Check sheet for the modelled part. Datum: model origin and axes. Units: mm. A direction names the side the tool comes from. Give positions to 0.01 mm unless a question says otherwise; leave off trailing zeros. Order: outer loops, then holes, each group sorted by start corner. A loop starts at its lowest first (then second) coordinate and runs counter-clockwise, first axis right, second up. Notation, with made-up numbers: (75, -1.5) - (97, -1.5) arc R29 ccw to (97, 34.5) - close; hole circle Ø1 at (62, 65.25). An arc over 180 degrees is marked (long way). Answer in a Markdown table with one row per item.
from build123d import *

# Parameters (mm, degrees)
SKETCH1_W                     = 60
SKETCH1_H                     = 60
BOSS_EXTRUDE1_DEPTH           = 10
SKETCH1_3_W                   = 9.5
SKETCH1_3_H                   = 10
BOSS_EXTRUDE2_DEPTH           = 20
BOSS_EXTRUDE3_START           = -10
SKETCH1_4_W                   = 34.6
SKETCH1_4_H                   = 60
BOSS_EXTRUDE3_DEPTH           = 22.5
CBORE_FOR_M3_SHCS1_AT_2_COUNT = 2
CBORE_FOR_M3_SHCS1_AT_2_PITCH = 40
SKETCH6_R                     = 2.25
CUT_EXTRUDE1_DEPTH            = 10
FILLET1_R                     = 1


with BuildPart() as part:
    # Sketch1 → Boss-Extrude1 (new body)
    with BuildSketch(Plane(origin=(0, 0, 0), x_dir=(1, 0, 0), z_dir=(0, 1, 0))):
        Rectangle(SKETCH1_W, SKETCH1_H)
    extrude(amount=-BOSS_EXTRUDE1_DEPTH)

    # Sketch1<3> → Boss-Extrude2 (add)
    with BuildSketch(Plane(origin=(0, 0, 0), x_dir=(1, 0, 0), z_dir=(0, 1, 0))):
        with Locations((-25.25, -15.65)):
            Rectangle(SKETCH1_3_W, SKETCH1_3_H)
        with Locations((25.25, -15.65)):
            Rectangle(SKETCH1_3_W, SKETCH1_3_H)
    extrude(amount=BOSS_EXTRUDE2_DEPTH)

    # Sketch1<4> → Boss-Extrude3 (add)
    with BuildSketch(Plane(origin=(0, 0, 0), x_dir=(1, 0, 0), z_dir=(0, 1, 0)).offset(BOSS_EXTRUDE3_START)):
        with Locations((12.7, 0)):
            Rectangle(SKETCH1_4_W, SKETCH1_4_H)
    extrude(amount=-BOSS_EXTRUDE3_DEPTH)

    # Sketch3 → CBORE for M3 SHCS1 (revolve, cut)
    with BuildSketch(Plane(origin=(30, -23.49, 20), x_dir=(0, 0, -1), z_dir=(0, 1, 0))):
        Polygon((0, 0), (0, 35.681549114), (1.8, 34.6), (1.8, 23), (3.25, 23), (3.25, 0.025), (3.275, 0), align=None)
    cbore_for_m3_shcs1 = revolve(axis=Axis((36.35, -23.49, 20), (-1, 0, 0)), mode=Mode.SUBTRACT)

    # CBORE for M3 SHCS1 at 2: CBORE for M3 SHCS1 ×2
    with Locations(*[(0, 0, -i * CBORE_FOR_M3_SHCS1_AT_2_PITCH) for i in range(1, CBORE_FOR_M3_SHCS1_AT_2_COUNT)]):
        add(cbore_for_m3_shcs1, mode=Mode.SUBTRACT)

    # Sketch5 → CBORE for M3 SHCS2 (revolve, cut)
    with BuildSketch(Plane(origin=(-18.09, 0, -20), x_dir=(0, 0, 1), z_dir=(1, 0, 0))):
        Polygon((0, 0), (0, 11.081549114), (1.8, 10), (1.8, 3), (3.25, 3), (3.25, 0.025), (3.275, 0), align=None)
    revolve(axis=Axis((-18.09, 6.35, -20), (0, -1, 0)), mode=Mode.SUBTRACT)

    # Sketch6 → Cut-Extrude1 (cut)
    with BuildSketch(Plane.XY.offset(20.65)):
        with Locations((-23.725, 15)):
            Circle(SKETCH6_R)
        with Locations((-23.725, 5)):
            Circle(SKETCH6_R)
        with Locations(Location((23.725, 5, 0), (0, 0, 180))):
            Circle(SKETCH6_R)
        with Locations(Location((23.725, 15, 0), (0, 0, 180))):
            Circle(SKETCH6_R)
    extrude(amount=-CUT_EXTRUDE1_DEPTH, mode=Mode.SUBTRACT)

    # Fillet1
    fillet1_edges = [part.edges().sort_by_distance(p)[0] for p in [
        (-17.3, -10, -30),
        (-30, -10, 0),
        (-30, 0, 25.325),
        (-25.25, 20, 20.65),
        (-30, 10, 20.65),
        (-20.5, 20, 15.65),
        (-25.25, 20, 10.65),
        (-30, 10, 10.65),
        (-30, 20, 15.65),
        (-25.25, 0, 20.65),
        (-25.25, 0, 10.65),
        (30, 0, 25.325),
        (30, 20, 15.65),
        (30, 10, 20.65),
        (25.25, 0, 10.65),
        (30, 10, 10.65),
        (25.25, 0, 20.65),
        (25.25, 20, 10.65),
        (20.5, 20, 15.65),
        (25.25, 20, 20.65),
        (-17.3, -10, 30),
        (-4.6, -32.5, 0),
        (-4.6, -21.25, 30),
        (-4.6, -21.25, -30),
        (12.7, -32.5, -30),
        (30, -32.5, 0),
        (12.7, -32.5, 30),
        (0, 0, 30),
        (-30, 0, -9.675),
        (0, 0, -30),
        (30, 0, -9.675),
        (30, -16.25, 30),
        (-30, -5, 30),
        (-30, -5, -30),
        (30, -16.25, -30),
    ]]
    fillet(fillet1_edges, radius=FILLET1_R)


solid = part.part
(1) Cross-section at B-B, the plane y = -23.49. Record the cut outline in (x, z) (3 decimals), then the cut area to 3 significant figures.
Geometry says:
| item | result |
|---|---|
| outline | (-4.6, -29) arc R1 ccw to (-3.6, -30) - (29, -30) arc R1 ccw to (30, -29) - (30, -23.275) - (29.975, -23.25) - (7, -23.25) - (7, -21.8) - (-4.6, -21.8) - close; (-4.6, -18.2) - (7, -18.2) - (7, -16.75) - (29.975, -16.75) - (30, -16.725) - (30, 16.725) - (29.975, 16.75) - (7, 16.75) - (7, 18.2) - (-4.6, 18.2) - close; (-4.6, 21.8) - (7, 21.8) - (7, 23.25) - (29.975, 23.25) - (30, 23.275) - (30, 29) arc R1 ccw to (29, 30) - (-3.6, 30) arc R1 ccw to (-4.6, 29) - close |
| area | 1,690 mm² |
(2) Mould release check, pull along Z, two halves, no side actions. Record for faces 5 (the cylindrical face through (18.648, -23.633, 23.247)), 6 (the flat face through (-17, -10, 0)), 7 (the flat face through (-25, 10, 20.65)): pulls with the +Z half, pulls with the -Z half, needs draft (parallel to the pull), parting line crosses it, or undercut.
Geometry says:
| item | result |
|---|---|
| face 5 | undercut |
| face 6 | needs draft |
| face 7 | pulls with the +Z half |
(3) Cross-section at A-A, the plane z = -20. Give the number of separate pieces and of enclosed holes in the cut face, then the cut area to 3 significant figures.
Geometry says:
| item | result |
|---|---|
| separate pieces | 3 |
| enclosed holes | 0 |
| area | 1,140 mm² |
(4) Access from +Z, -Z, +X, -X, +Y, -Y to the whole of each face (thin tool, end or side, straight path). Record for faces 1 (the flat face through (-4.6, -21, 0)), 2 (the cylindrical face through (-20.287, -1.492, -22.395)), 3 (the flat face through (-20.5, 9, 16)), 4 (the flat face through (7, -22.1, -18.6)).
Geometry says:
| item | result |
|---|---|
| face 1 | +Z, -Z, -X, -Y |
| face 2 | +Y |
| face 3 | +Z, -Z, +Y |
| face 4 | +X |
(5) Thickness scan on L1, parallel to Z at x = 3.5, y = -23.49; L2, parallel to Z at x = 18.75, y = -23.49; L3, parallel to Y at x = -16.5, z = 3.5. Record the ranges inside material, lowest first.
Geometry says:
| item | result |
|---|---|
| L1 | -30 to -21.8, -18.2 to 18.2, 21.8 to 30 |
| L2 | -30 to -23.25, -16.75 to 16.75, 23.25 to 30 |
| L3 | -10 to 0 |
(6) Gauge pin test, flat ends, axial feed: P1, Ø2, axis at x = -18.5, z = -21, coming from the +Y side; P2, Ø8.5, axis at y = -23.49, z = -20, coming from the -X side; P3, Ø4, axis at x = -16, z = -3.5, coming from the -Y side; P4, Ø3, axis at y = -23.5, z = -20, coming from the +X side. Record the tip position at first contact, or that the pin passes through.
Geometry says:
| item | result |
|---|---|
| P1 | y = -3 |
| P2 | x = -4.6 |
| P3 | y = -10 |
| P4 | through |
(7) Cross-section at C-C, the plane z = 13. Record the cut outline in (x, y) (3 decimals).
Geometry says:
| item | result |
|---|---|
| outline | (-30, -9) arc R1 ccw to (-29, -10) - (-4.6, -10) - (-4.6, -31.5) arc R1 ccw to (-3.6, -32.5) - (29, -32.5) arc R1 ccw to (30, -31.5) - (30, 19) arc R1 ccw to (29, 20) - (21.5, 20) arc R1 ccw to (20.5, 19) - (20.5, 0) - (-20.5, 0) - (-20.5, 19) arc R1 ccw to (-21.5, 20) - (-29, 20) arc R1 ccw to (-30, 19) - close; hole circle Ø4.5 at (-23.725, 5); hole circle Ø4.5 at (-23.725, 15); hole circle Ø4.5 at (23.725, 5); hole circle Ø4.5 at (23.725, 15) |
(8) Cross-section at D-D, the plane x = 4. Record the cut outline in (y, z), then the cut area to 3 significant figures.
Geometry says:
| item | result |
|---|---|
| outline | (-32.5, -29) arc R1 ccw to (-31.5, -30) - (-1, -30) arc R1 ccw to (0, -29) - (0, 29) arc R1 ccw to (-1, 30) - (-31.5, 30) arc R1 ccw to (-32.5, 29) - close; hole circle Ø3.6 at (-23.49, -20); hole circle Ø3.6 at (-23.49, 20) |
| area | 1,930 mm² |
